Geometry: final body of the model. Coordinates: model frame, mm. A direction names the side the tool comes from. Round coordinates to 2 decimals unless told otherwise and drop trailing zeros. Loops run counter-clockwise (first coordinate to the right, second up) from the corner with the lowest first, then second, coordinate; pieces in that order, holes last. Notation, with made-up numbers: (29.25, 23.5) - (73.25, 23.5) arc R20 cw to (73.25, 33.5) - close; hole circle Ø3 at (85.5, 3). An arc over 180 degrees is marked (long way). Return JSON: item names as keys, results as strings. Group by question number.
1. Section C-C on x = 155. Return loops of the section in (y, z), and give its area (4 significant figures).
2. Draft query along Y for faces 4 (the face through (17, 26, 50)), 5 (the face through (181, 300, 7)), 6 (the face through (110, 45, 7)). Return one class per face: +Y half, -Y half, draft (parallel to the pull), parting line (faces both ways), or undercut.
3. Section B-B on x = 124.5. Return loops of the section in (y, z).
4. First-contact query: pin 1 Ø4.5 at (x, z) = (158, 9.5) entering from -Y; pin 2 Ø4 at (x, y) = (57.5, 58) entering from +Z. Flat tips, straight axial feed; report the tip coordinate or a pass-through.
5. Set-up query: faces 1 (the face through (87, 25, 14)), 2 (the face through (9.86, 50.49, 45.72)), 3 (the face through (207, 164, 15)). Return all of +Z, -Z, +X, -X, +Y, -Y with unobstructed straight access to the full face (end or side cutting, diameter ignored); none if empty.
6. Section A-A on y = 196. Return loops of the section in (x, z), and give its area (3 significant figures).
7. Material intervals for probe 1 along Y at (x, z) = (155, 4.75); probe 2 along X at (y, z) = (275, 8.5); probe 3 along X at (y, z) = (118, 7), sorted ascending.
8. Section D-D on z = 40.5. Return loops of the section in (x, y).
from build123d import *

# Parameters (mm, degrees)
F0_R     = 7
F1_DEPTH = 15
F2_DEPTH = 50
F3_W     = 220
F3_H     = 30
F4_DEPTH = 25
F5_R     = 14.99999
F6_R     = 5


# Not quite as in the source:
# - a fillet or chamfer is up to 0.001 mm smaller than in the source, because OpenCascade refuses the exact size


with BuildPart() as f1:
    # F0 (on Top) → F1 (new body)
    with BuildSketch(Plane.XY):
        Polygon((0, 300), (0, 0), (60, 0), (60, 5), (5, 5), (5, 25), (20, 25), (20, 300), align=None)
        Polygon((80, 300), (20, 300), (20, 25), (220, 25), (220, 300), (140, 300), (145, 295), (75, 295), align=None)
        with Locations((65, 55)):
            Circle(F0_R, mode=Mode.SUBTRACT)
        with Locations((155, 55)):
            Circle(F0_R, mode=Mode.SUBTRACT)
        Polygon((40, 75), (40, 255), (85, 255), (85, 270), (135, 270), (135, 255), (200, 255), (200, 75), (135, 75), (135, 45), (85, 45), (85, 75), align=None, mode=Mode.SUBTRACT)
        with Locations((65, 275)):
            Circle(F0_R, mode=Mode.SUBTRACT)
        with Locations((155, 275)):
            Circle(F0_R, mode=Mode.SUBTRACT)
    extrude(amount=F1_DEPTH)

    # F0 (on Top) → F2 (join)
    with BuildSketch(Plane.XY):
        Polygon((0, 300), (0, 0), (60, 0), (60, 5), (5, 5), (5, 25), (20, 25), (20, 300), align=None)
    extrude(amount=F2_DEPTH)

    # F3 (on face) → F4 (cut)
    with BuildSketch(Plane.YZ.offset(20)):
        with Locations((165, 35)):
            Rectangle(F3_W, F3_H)
    extrude(amount=-F4_DEPTH, mode=Mode.SUBTRACT)

    # F5 (radius 15 in the source; OpenCascade refuses exactly that, so slightly less here)
    f5_edges = [f1.edges().sort_by_distance(p)[0] for p in [
        (10, 275, 20),
        (10, 55, 20),
        (10, 275, 50),
        (10, 55, 50),
    ]]
    fillet(f5_edges, radius=F5_R)

    # F6
    f6_edges = [f1.edges().sort_by_distance(p)[0] for p in [
        (85, 75, 7.5),
        (135, 75, 7.5),
        (85, 45, 7.5),
        (135, 45, 7.5),
        (85, 255, 7.5),
        (85, 270, 7.5),
        (135, 255, 7.5),
        (135, 270, 7.5),
        (40, 75, 7.5),
        (40, 255, 7.5),
        (200, 255, 7.5),
        (200, 75, 7.5),
    ]]
    fillet(f6_edges, radius=F6_R)


solid = f1.part
Taken from the geometry:
{
 "1": {"outline": "(25, 0) - (48, 0) - (48, 15) - (25, 15) - close; (62, 0) - (75, 0) - (75, 15) - (62, 15) - close; (255, 0) - (268, 0) - (268, 15) - (255, 15) - close; (282, 0) - (300, 0) - (300, 15) - (282, 15) - close", "area": "1,005 mm2"},
 "2": {"face 4": "draft", "face 5": "+Y half", "face 6": "undercut"},
 "3": {"outline": "(25, 0) - (45, 0) - (45, 15) - (25, 15) - close; (270, 0) - (295, 0) - (295, 15) - (270, 15) - close"},
 "4": {"pin 1": "y = 25", "pin 2": "z = 15"},
 "5": {"face 1": "+Z, -Z, +X", "face 2": "+Z, +X, -X", "face 3": "+Z, +X, +Y"},
 "6": {"outline": "(0, 0) - (40, 0) - (40, 15) - (20, 15) - (20, 20) - (0, 20) - close; (200, 0) - (220, 0) - (220, 15) - (200, 15) - close", "area": "1,000 mm2"},
 "7": {"probe 1": "25 to 48, 62 to 75, 255 to 268, 282 to 300", "probe 2": "0 to 58, 72 to 148, 162 to 220", "probe 3": "0 to 40, 200 to 220"},
 "8": {"outline": "(0, 0) - (60, 0) - (60, 5) - (5, 5) - (5, 25) - (20, 25) - (20, 53.96) - (0, 53.96) - close; (0, 276.04) - (20, 276.04) - (20, 300) - (0, 300) - close"}
}
